Autodesk Inventor part; units mm, degrees
ref_plane "YZ Plane" through (0, 0, 0) normal (1, 0, 0) x (0, 1, 0)
ref_plane "XZ Plane" through (0, 0, 0) normal (0, 1, 0) x (-1, 0, 0)
ref_plane "XY Plane" through (0, 0, 0) normal (0, 0, 1) x (1, 0, 0)
sketch "Sketch1" plane through (0, 0, 0) normal (0, 0, 1) x (1, 0, 0)
  line L0 (-10.3124, -6.4135) -> (10.3124, -6.4135)
  line L1 (10.3124, -6.4135) -> (10.3124, 6.4135) construction
  line L2 (10.3124, 6.4135) -> (-10.3124, 6.4135)
  line L3 (-10.3124, 6.4135) -> (-10.3124, -6.4135) construction
  line L4 (-10.3124, -6.4135) -> (10.3124, 6.4135) construction
  line L5 (10.3124, -6.4135) -> (-10.3124, 6.4135) construction
  arc A0 (10.3124, -6.4135) -> (10.3124, 6.4135) centre (4.1562, 0) ccw
  arc A1 (-10.3124, 6.4135) -> (-10.3124, -6.4135) centre (-1.4224, 0) ccw
  point P0 (0, 0)
  dimension "d0" = 12.827
  dimension "d1" = 8.89
  dimension "d2" = 8.89
  dimension "d3" = 1.4224
extrude "Extrusion1" add sketch "Sketch1" along normal blind 3.175
sketch "Sketch2" plane through (0, 0, 0) normal (0, 0, -1) x (-1, 0, 0)
  circle A0 centre (0, 0) radius 3.175
  dimension "d6" = 6.35
extrude "Extrusion2" cut sketch "Sketch2" against normal blind 5.08
sketch "Sketch3" plane through (0, 0, 3.175) normal (0, 0, 1) x (1, 0, 0)
  circle A0 centre (0, 0) radius 3.175
  circle A1 centre (0, 0) radius 3.556
  dimension "d9" = 7.112
extrude "Extrusion3" add sketch "Sketch3" along normal blind 1.27
thread "Thread1"
equation "\"d2\" = d1"
properties part number "3786_economy_slide_tnuts"
Work out the finished part from the listing and answer in its coordinate system (mm). A direction names the side the tool comes from. Give positions to 0.01 mm unless a question says otherwise; leave off trailing zeros. Loops run counter-clockwise (first coordinate to the right, second up) from the corner with the lowest first, then second, coordinate; pieces in that order, holes last. Notation, with made-up numbers: (-30.75, 63.25) -> (19.25, 63.25) arc R9 cw to (19.25, 79.25) -> close; hole circle Ø6 at (89, -19). An arc over 180 degrees is marked (long way). Use CSV: the item, a comma, the result in double quotes.
1. The part is cut by section D-D (x = -8.25). Write down the section's boundary in (y, z) (1 decimal), then the cut area to 3 significant figures.
Found:
outline,"(-6.4, 0) -> (6.4, 0) -> (6.4, 3.2) -> (-6.4, 3.2) -> close"
area,"40.7 mm^2"
2. Straight lines are drawn through the part: line 1 (X direction, y = 0, z = 1.4) (3 decimals); line 2 (Y direction, x = 0, z = 3.8) (3 decimals); line 3 (Z direction, x = 2.75, y = -2.5) (3 decimals). For each, find the intervals that lie inside material, in ascending order.
Found:
line 1,"-12.384 to -3.175, 3.175 to 13.046"
line 2,"-3.556 to -3.175, 3.175 to 3.556"
line 3,"0 to 3.175"
3. The part is cut by section A-A (y = 0). Write down the section's boundary in (x, z) (3 decimals), then the cut area to 3 significant figures.
Found:
outline,"(-12.384, 0) -> (-3.175, 0) -> (-3.175, 4.445) -> (-3.556, 4.445) -> (-3.556, 3.175) -> (-12.384, 3.175) -> close; (3.175, 0) -> (13.046, 0) -> (13.046, 3.175) -> (3.556, 3.175) -> (3.556, 4.445) -> (3.175, 4.445) -> close"
area,"61.5 mm^2"
4. A tool of negligible diameter and unlimited length cuts with its end or side. For faces 1 (the cylindrical face through (-0.77, 3.47, 3.8)), 2 (the flat face through (0, -6.414, 2)), from which of +Z, -Z, +X, -X, +Y, -Y can it reach the whole face along a straight path? Write none if from no direction.
Found:
face 1,"+Z"
face 2,"+Z, -Z, +X, -X, -Y"
5. Flat-ended cylindrical pins translate along their axes: pin 1 Ø3 at (x, y) = (-3, -2.5) entering from +Z (3 decimals); pin 2 Ø2 at (y, z) = (-1.5, 3) entering from -X. Find the tip coordinate at first contact, or state that the pin passes through.
Found:
pin 1,"z = 4.445"
pin 2,"x = -12.37"
